```python
from build123d import *

# Parameters (mm, degrees)
F0_W     = 204.5249342918
F0_H     = 195.493966341
F1_DEPTH = 2.54
F3_DEPTH = 2.8448


with BuildPart() as f1:
    # F0 (on Top) → F1 (new body)
    with BuildSketch(Plane.XY):
        with Locations((2.9734447598, 3.9486810565)):
            Rectangle(F0_W, F0_H)
    extrude(amount=F1_DEPTH)

    # F2 (on face) → F3 (join)
    with BuildSketch(Plane.XY.offset(2.54)):
        with BuildLine():
            Line((-17.3801127821, -43.1336462498), (-17.3801127821, -93.798302114))
            Line((-17.3801127821, -93.798302114), (17.8944449872, -93.798302114))
            Line((17.8944449872, -93.798302114), (17.8944449872, -43.8535362482))
            add(Edge.make_bspline(
                [(17.8944449872, -43.8535362482), (19.6377973848, -40.8099152189), (23.1994125002, -34.5918914397), (22.8672950733, -22.568415978), (24.6099326679, -16.2696792332), (27.280489177, -8.681472684), (34.7377245339, -4.0405072298), (40.9514398387, -4.4219057306), (44.1720969975, -4.6195900068)],
                knots=[0, 0, 0, 0, 0.1822465719, 0.3723241188, 0.5162955376, 0.6700276511, 0.828970631, 1, 1, 1, 1], degree=3))
            Line((44.1720969975, -4.6195900068), (105.2359119058, -4.6195900068))
            Line((105.2359119058, -4.6195900068), (105.2359119058, 12.6577429473))
            Line((105.2359119058, 12.6577429473), (36.2526699901, 12.6577429473))
            Line((36.2526699901, 12.6577429473), (29.0531925857, 12.6577429473))
            add(Edge.make_bspline(
                [(29.0531925857, 12.6577429473), (26.7554854749, 12.3173098622), (22.0675905119, 11.6227415521), (18.5421925524, 15.1794504397), (16.7447198182, 16.992887482)],
                knots=[0, 0, 0, 0, 0.4901362187, 1, 1, 1, 1], degree=3))
            Line((16.7447198182, 16.992887482), (16.7447198182, 101.695664227))
            Line((16.7447198182, 101.695664227), (-17.3801127821, 101.695664227))
            Line((-17.3801127821, 101.695664227), (-17.3801127821, -43.1336462498))
        make_face()
    extrude(amount=F3_DEPTH)


solid = f1.part
```
Source: CAD feature listing. Evaluate the final solid. Frame: model axes, mm. A direction names the side the tool comes from. Round coordinates to 2 decimals unless told otherwise and drop trailing zeros. Write each loop counter-clockwise with the first axis right and the second up, starting at its lowest first coordinate (ties: lowest second). Pieces come first, ordered by that corner, then holes. Notation, with made-up numbers: M 85,88.25 L 135,88.25 A25 cw 135,118.25 Z; hole C 29,16 d7. An arc over 180 degrees is marked long. Use CSV: the item, a comma, the result in double quotes. Start each with the question number.
Q1. Line query: line 1 (X direction, y = 82, z = 4.55); line 2 (Z direction, x = -55, y = -24); line 3 (X direction, y = -0.5, z = 4.7). Output: solid intervals per line, ascending. Write a range as from..to.
Q2. Access query for faces 1 (the face through (-59, 5, 2.54)), 2 (the face through (61, -48, 2.54)), 3 (the face through (60, 57, 2.54)), 4 (the face through (2, 101.696, 1)). Directions: +Z, -Z, +X, -X, +Y, -Y. A direction counts if a zero-diameter tool reaches every point of the face in a straight line with its end or side. Return the directions, or none.
Q3. Cut plane A-A on x = 74.5. Output: boundary loops of the cut face in (y, z), plus the area to 3 significant figures.
Q4. First-contact query: P1, Ø3, axis at x = 86.5, z = 4.5, coming from the -Y side; P2, Ø2.5, axis at y = -81, z = 4.5, coming from the +X side; P3, Ø1, axis at x = -41.5, y = 60, coming from the -Z side; P4, Ø6, axis at x = 77.5, y = 67, coming from the +Z side. Flat tips, straight axial feed; report the tip coordinate or a pass-through.
Q5. Cut plane B-B on y = -52. Output: boundary loops of the cut face in (x, z), plus the area to 3 significant figures.
Results found:
1,line 1,"-17.38..16.74"
1,line 2,"0..2.54"
1,line 3,"-17.38..105.24"
2,face 1,"+Z, -X, +Y, -Y"
2,face 2,"+Z, +X, -Y"
2,face 3,"+Z, +X, +Y"
2,face 4,"+Z, -Z, +X, -X, +Y"
3,outline,"M -93.8,0 L 101.7,0 L 101.7,2.54 L 12.66,2.54 L 12.66,5.38 L -4.62,5.38 L -4.62,2.54 L -93.8,2.54 Z"
3,area,"546 mm^2"
4,P1,"y = -4.62"
4,P2,"x = 17.89"
4,P3,"z = 0"
4,P4,"z = 2.54"
5,outline,"M -99.29,0 L 105.24,0 L 105.24,2.54 L 17.89,2.54 L 17.89,5.38 L -17.38,5.38 L -17.38,2.54 L -99.29,2.54 Z"
5,area,"620 mm^2"
